from build123d import *

# Parameters (mm, degrees)
SKETCH1_W           = 25.4
SKETCH1_H           = 25.4
SKETCH1_W_2         = 22.225
SKETCH1_H_2         = 22.225
BOSS_EXTRUDE1_DEPTH = 152.4
SKETCH4_R           = 2.54
CUT_EXTRUDE3_DEPTH  = 157.576115675


with BuildPart() as part:
    # Sketch1 → Boss-Extrude1 (new body)
    with BuildSketch(Plane.XY):
        with Locations((12.7, 12.7)):
            Rectangle(SKETCH1_W, SKETCH1_H)
        with Locations((12.7, 12.7)):
            Rectangle(SKETCH1_W_2, SKETCH1_H_2, mode=Mode.SUBTRACT)
    extrude(amount=BOSS_EXTRUDE1_DEPTH)

    # Sketch4 → Cut-Extrude3 (cut, through all)
    with BuildSketch(Plane(origin=(25.4, 0, 0), x_dir=(0, 0, -1), z_dir=(1, 0, 0))):
        with Locations((-139.7, 12.7)):
            Circle(SKETCH4_R)
        with Locations((-114.3, 12.7)):
            Circle(SKETCH4_R)
        with Locations((-88.9, 12.7)):
            Circle(SKETCH4_R)
        with Locations(Location((-63.5, 12.7, 0), (0, 0, 180))):
            Circle(SKETCH4_R)
        with Locations(Location((-38.1, 12.7, 0), (0, 0, 180))):
            Circle(SKETCH4_R)
        with Locations(Location((-12.7, 12.7, 0), (0, 0, 180))):
            Circle(SKETCH4_R)
    extrude(amount=-CUT_EXTRUDE3_DEPTH, mode=Mode.SUBTRACT)


solid = part.part
Geometry check sheet. Reference: the model listing, model coordinates, mm. A direction names the side the tool comes from. Give positions to 0.01 mm unless a question says otherwise; leave off trailing zeros. Write each loop counter-clockwise with the first axis right and the second up, starting at its lowest first coordinate (ties: lowest second). Pieces come first, ordered by that corner, then holes. Notation, with made-up numbers: M 78.25,65 L 111.25,65 A32 ccw 111.25,91 Z; hole C -39.75,-24.5 d8. An arc over 180 degrees is marked long. One line per question, with ' | ' between items.
1. Mould release check, pull along Y, two halves, no side actions. Record for faces 1 (the face through (0, 13, 75)), 2 (the face through (13, 0, 75)), 3 (the face through (24.617, 12.812, 142.238)): released by +Y, released by -Y, zero draft, split by the parting line, or undercut.
Ans:
face 1: zero draft | face 2: released by -Y | face 3: undercut
2. Scan lines: line 1 along X through (y, z) = (23.25, 124); line 2 along Y through (x, z) = (1.15, 38.1). Record each from-to range of solid material in increasing order. Write a range as from..to.
Ans:
line 1: 0..1.59, 23.81..25.4 | line 2: 0..10.16, 15.24..25.4
3. Cross-section at A-A (y = 21.5). Enter the section's corners in (x, z).
Ans:
outline: M 0,0 L 1.59,0 L 1.59,152.4 L 0,152.4 Z; M 23.81,0 L 25.4,0 L 25.4,152.4 L 23.81,152.4 Z
4. Cross-section at B-B (z = 72.5). Enter the section's corners in (x, y).
Ans:
outline: M 0,0 L 25.4,0 L 25.4,25.4 L 0,25.4 Z; hole M 1.59,1.59 L 23.81,1.59 L 23.81,23.81 L 1.59,23.81 Z
5. Cross-section at D-D (z = 114.3). Enter the section's corners in (x, y).
Ans:
outline: M 0,0 L 25.4,0 L 25.4,10.16 L 23.81,10.16 L 23.81,1.59 L 1.59,1.59 L 1.59,10.16 L 0,10.16 Z; M 0,15.24 L 1.59,15.24 L 1.59,23.81 L 23.81,23.81 L 23.81,15.24 L 25.4,15.24 L 25.4,25.4 L 0,25.4 Z
6. Set-up check for faces 4 (the face through (24.62, 14.42, 116.17)), 5 (the face through (13, 23.812, 75)): record each of +Z, -Z, +X, -X, +Y, -Y from which the full face is reachable in a straight line by a thin tool's end or side.
Ans:
face 4: +X, -X | face 5: +Z, -Z
